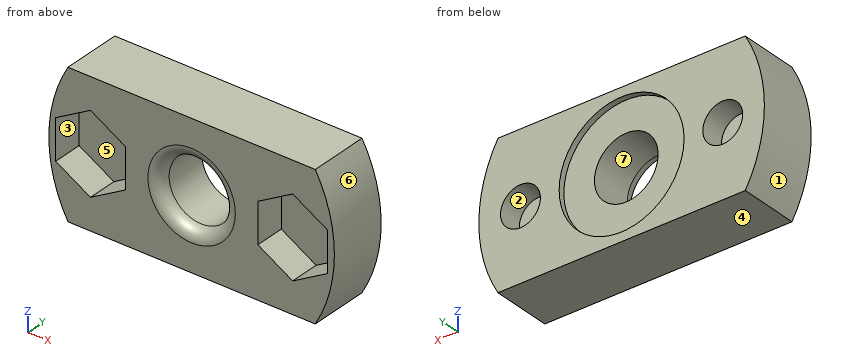
```python
from build123d import *

# Parameters (mm, degrees)
SKETCH1_R           = 12
SKETCH1_R_2         = 2.675
BOSS_EXTRUDE1_DEPTH = 5
SKETCH3_R           = 1.675
CUT_EXTRUDE1_DEPTH  = 6
CUT_EXTRUDE2_DEPTH  = 2.5
CUT_EXTRUDE4_DEPTH  = 10
FILLET1_R           = 1
SKETCH7_R           = 5.25
CUT_EXTRUDE5_DEPTH  = 0.5
SKETCH8_R           = 1.675
BOSS_EXTRUDE2_DEPTH = 0.5


with BuildPart() as part:
    # Sketch1 → Boss-Extrude1 (new body)
    with BuildSketch(Plane(origin=(0, 0, 0), x_dir=(1, 0, 0), z_dir=(0, 1, 0))):
        Circle(SKETCH1_R)
        Circle(SKETCH1_R_2, mode=Mode.SUBTRACT)
    extrude(amount=BOSS_EXTRUDE1_DEPTH)

    # Sketch3 → Cut-Extrude1 (cut)
    with BuildSketch(Plane(origin=(0, 5, 0), x_dir=(1, 0, 0), z_dir=(0, 1, 0))):
        with Locations((-8.5, 0)):
            Circle(SKETCH3_R)
        with Locations((8.5, 0)):
            Circle(SKETCH3_R)
    extrude(amount=-CUT_EXTRUDE1_DEPTH, mode=Mode.SUBTRACT)

    # Sketch4 → Cut-Extrude2 (cut)
    with BuildSketch(Plane.XZ):
        Polygon((-11.425, -1.688749537), (-8.5, -3.377499075), (-5.575, -1.688749537), (-5.575, 1.688749537), (-8.5, 3.377499075), (-11.425, 1.688749537), align=None)
        Polygon((11.425, 1.688749537), (11.425, -1.688749537), (8.5, -3.377499075), (5.575, -1.688749537), (5.575, 1.688749537), (8.5, 3.377499075), align=None)
    extrude(amount=-CUT_EXTRUDE2_DEPTH, mode=Mode.SUBTRACT)

    # Sketch6 → Cut-Extrude4 (cut)
    with BuildSketch(Plane.XZ):
        with BuildLine():
            Line((-10.392304845, 6), (10.392304845, 6))
            ThreePointArc((10.392304845, 6), (0, 12), (-10.392304845, 6))
        make_face()
        with BuildLine():
            Line((-10.392304845, -6), (10.392304845, -6))
            ThreePointArc((10.392304845, -6), (0, -12), (-10.392304845, -6))
        make_face()
    extrude(amount=-CUT_EXTRUDE4_DEPTH, mode=Mode.SUBTRACT)

    # Fillet1
    fillet1_edges = [part.edges().sort_by_distance(p)[0] for p in [
        (-2.675, 0, 0),
    ]]
    fillet(fillet1_edges, radius=FILLET1_R)

    # Sketch7 → Cut-Extrude5 (cut)
    with BuildSketch(Plane(origin=(0, 5, 0), x_dir=(1, 0, 0), z_dir=(0, 1, 0))):
        Circle(SKETCH7_R)
    extrude(amount=-CUT_EXTRUDE5_DEPTH, mode=Mode.SUBTRACT)

    # Sketch8 → Boss-Extrude2 (add)
    with BuildSketch(Plane.XZ.offset(-2.5)):
        with Locations((8.5, 0)):
            Circle(SKETCH8_R)
        with Locations((-8.5, 0)):
            Circle(SKETCH8_R)
    extrude(amount=-BOSS_EXTRUDE2_DEPTH)


solid = part.part
```
Model file for the job. Use its own axes, mm. Face numbers are marked on the shaded views. A direction names the side the tool comes from. Give positions to 0.01 mm unless a question says otherwise; leave off trailing zeros. Loops run counter-clockwise (first coordinate to the right, second up) from the corner with the lowest first, then second, coordinate; pieces in that order, holes last. Notation, with made-up numbers: M 73,-36.5 L 104,-36.5 A17 cw 104,-16.5 Z; hole C -22,70.5 d11. An arc over 180 degrees is marked long. Use one line per item in the form item = value.
Item 1: Two-plate mould, pull along X, no slides. Class the marked faces 4, 5, 6 and 7: released by +X, released by -X, zero draft, split by the parting line, or undercut.
Filled in:
face_4 = zero draft
face_5 = undercut
face_6 = released by +X
face_7 = undercut
Item 2: Slice it at D-D on z = 4.5. List the corners of the cut face in (x, y), and give its area (3 significant figures).
Filled in:
outline = M -11.12,0 L 11.12,0 L 11.12,5 L 2.7,5 L 2.7,4.5 L -2.7,4.5 L -2.7,5 L -11.12,5 Z
area = 109 mm^2
Item 3: Slice it at C-C on y = 3.4. List the corners of the cut face in (x, z) (3 decimals).
Filled in:
outline = M -10.392,-6 L 10.392,-6 A12 ccw 10.392,6 L -10.392,6 A12 ccw Z; hole C -8.5,0 d3.35; hole C 0,0 d5.35; hole C 8.5,0 d3.35
Item 4: Which spindle directions (+Z, -Z, +X, -X, +Y, -Y) get a long thin tool onto all of the face, cutting with end or side? Do the marked faces 1, 2 and 3. Say none if no direction does.
Filled in:
face_1 = -X, +Y, -Y
face_2 = +Y
face_3 = -Y
Item 5: Slice it at A-A on x = 0. List the corners of the cut face in (y, z) (3 decimals).
Filled in:
outline = M 0,-6 L 5,-6 L 5,-5.25 L 4.5,-5.25 L 4.5,-2.675 L 1,-2.675 A1 ccw 0,-3.675 Z; M 0,3.675 A1 ccw 1,2.675 L 4.5,2.675 L 4.5,5.25 L 5,5.25 L 5,6 L 0,6 Z
Item 6: Drill centre lines: L1, parallel to X at y = 3.7, z = 0 (3 decimals); L2, parallel to Z at x = -8.5, y = 4.3 (3 decimals); L3, parallel to Z at x = 0, y = 1.8 (3 decimals). Where is each one in solid material? Low to high.
Filled in:
L1 = -12 to -10.175, -6.825 to -2.675, 2.675 to 6.825, 10.175 to 12
L2 = -6 to -1.675, 1.675 to 6
L3 = -6 to -2.675, 2.675 to 6
Item 7: Flat gauge pins, fed straight in: pin 1 Ø1.8 at (x, z) = (7.5, -1.5) entering from -Y; pin 2 Ø3 at (x, z) = (-1.5, 1.5) entering from +Y; pin 3 Ø1.7 at (x, z) = (-8, 0.5) entering from +Y. Where does each tip first touch, or does it go through?
Filled in:
pin_1 = 2.5
pin_2 = 4.5
pin_3 = 3
